Part model, mm, in its own coordinate system. A direction names the side the tool comes from. Round coordinates to 2 decimals unless told otherwise and drop trailing zeros. Order: outer loops, then holes, each group sorted by start corner. A loop starts at its lowest first (then second) coordinate and runs counter-clockwise, first axis right, second up. Notation, with made-up numbers: (80, 87) -> (87, 87) arc R5 cw to (87, 96) -> close; hole circle Ø9 at (-20.5, -32). An arc over 180 degrees is marked (long way). Answer as a JSON object with one key per item and string values. Group by question number.
```python
from build123d import *

# Parameters (mm, degrees)
F0_W     = 106.8142578006
F0_H     = 34.0172816068
F0_W_2   = 91.846652329
F0_H_2   = 22.4514044821
F1_DEPTH = 25
F2_W     = 106.8142578006
F2_H     = 34.0172816068
F3_DEPTH = 3
F4_W     = 42.6840842701
F4_H     = 15.5962775201
F4_W_2   = 44.0205549821
F5_DEPTH = 42.7


with BuildPart() as f1:
    # F0 (on Front) → F1 (new body)
    with BuildSketch(Plane.XZ):
        with Locations((4.592332989, 0.3401720896)):
            Rectangle(F0_W, F0_H)
        with Locations((4.592332989, 0.6803460419)):
            Rectangle(F0_W_2, F0_H_2, mode=Mode.SUBTRACT)
    extrude(amount=F1_DEPTH)

    # F2 (on face) → F3 (join)
    with BuildSketch(Plane(origin=(0, 0, 0), x_dir=(-1, 0, 0), z_dir=(0, 1, 0))):
        with Locations((-4.592332989, 0.3401720896)):
            Rectangle(F2_W, F2_H)
    extrude(amount=F3_DEPTH)

    # F4 (on face) → F5 (cut)
    with BuildSketch(Plane.XY.offset(17.348812893)):
        with Locations((-27.4727537762, -4.79813876)):
            Rectangle(F4_W, F4_H)
        with Locations((35.9891843982, -4.79813876)):
            Rectangle(F4_W_2, F4_H)
    extrude(amount=-F5_DEPTH, mode=Mode.SUBTRACT)


solid = f1.part
```
Q1. Wall check: line 1 (Z direction, x = -34, y = -18); line 2 (X direction, y = -17, z = -6); line 3 (Y direction, x = -21, z = -11). Give the ranges that are in metal, low to high. Write a range as [from, to].
Q2. Band-saw the part on C-C (z = 7). List the corners of the cut face in (x, y), plus the area to 3 significant figures.
Q3. Band-saw the part on D-D (y = -9). List the corners of the cut face in (x, z), plus the area to 3 significant figures.
Q4. Two-plate mould, pull along X, no slides. Class faces 4 (the flat face through (4, 3, 1)), 5 (the flat face through (-48.815, -19, 0)), 6 (the flat face through (13.979, 0.3, 0.6)), 7 (the flat face through (4, -18, -10.545)): +X half, -X half, draft (parallel to the pull), parting line (faces both ways), or undercut.
Q5. Band-saw the part on B-B (y = -20.25). List the corners of the cut face in (x, z).
Q6. Which spindle directions (+Z, -Z, +X, -X, +Y, -Y) get a long thin tool onto all of the face, cutting with end or side? Do faces 1 (the flat face through (36, -12.596, -11)), 2 (the flat face through (-42, -12.596, 1)), 3 (the flat face through (-41.331, -19, 1)). Say none if no direction does.
Q7. Band-saw the part on A-A (x = -29). List the corners of the cut face in (y, z).
Q8. Drop flat-ended pins along their axis: pin 1 Ø1.5 at (x, y) = (-18, -10) entering from -Z; pin 2 Ø6 at (y, z) = (-7.5, 10) entering from +X; pin 3 Ø1 at (x, z) = (-30.5, -11.5) entering from +Y; pin 4 Ø6 at (x, z) = (0, -1) entering from -Y. Give the stop position or say it passes through.
Completed:
{
 "1": {"line 1": "[-16.67, -10.55], [11.91, 17.35]", "line 2": "[-48.81, -41.33], [50.52, 58]", "line 3": "[-25, -12.6]"},
 "2": {"outline": "(-48.81, -25) -> (-41.33, -25) -> (-41.33, -12.6) -> (-48.81, -12.6) -> close; (-6.13, 0) -> (13.98, 0) -> (13.98, 3) -> (-6.13, 3) -> close; (50.52, -25) -> (58, -25) -> (58, -12.6) -> (50.52, -12.6) -> close", "area": "246 mm2"},
 "3": {"outline": "(-6.13, -16.67) -> (13.98, -16.67) -> (13.98, -10.55) -> (-6.13, -10.55) -> close; (-6.13, 11.91) -> (13.98, 11.91) -> (13.98, 17.35) -> (-6.13, 17.35) -> close", "area": "233 mm2"},
 "4": {"face 4": "draft", "face 5": "-X half", "face 6": "+X half", "face 7": "undercut"},
 "5": {"outline": "(-48.81, -16.67) -> (58, -16.67) -> (58, 17.35) -> (-48.81, 17.35) -> close; hole (-41.33, -10.55) -> (50.52, -10.55) -> (50.52, 11.91) -> (-41.33, 11.91) -> close"},
 "6": {"face 1": "+Z, -Z, +X, +Y", "face 2": "+Z, -Z, -X, +Y", "face 3": "+Y, -Y"},
 "7": {"outline": "(-25, -16.67) -> (-12.6, -16.67) -> (-12.6, -10.55) -> (-25, -10.55) -> close; (-25, 11.91) -> (-12.6, 11.91) -> (-12.6, 17.35) -> (-25, 17.35) -> close"},
 "8": {"pin 1": "through", "pin 2": "x = 13.98", "pin 3": "y = -12.6", "pin 4": "y = 0"}
}
